Part model, mm, in its own coordinate system. A direction names the side the tool comes from. Give positions to 0.01 mm unless a question says otherwise; leave off trailing zeros. Write each loop counter-clockwise with the first axis right and the second up, starting at its lowest first coordinate (ties: lowest second). Pieces come first, ordered by that corner, then holes. Notation, with made-up numbers: (71.5, 53.5) - (98.5, 53.5) arc R26 ccw to (98.5, 89.5) - close; hole circle Ø3 at (-35, 15). An arc over 180 degrees is marked (long way). Answer in a Markdown table with one row per item. Add a question column.
1. Probe line 1 along Z through (x, y) = (-5.5, 11.5); line 2 along X through (y, z) = (11.5, 17.75); line 3 along X through (y, z) = (19, 14.5). List the from-to ranges inside material, lowest first.
2. Band-saw the part on A-A on x = 0. Write the cut outline in (y, z) (3 decimals), plus the area to 3 significant figures.
3. Pull direction Y, two halves, no side cores. Call faces 3 (the flat face through (-15.3, 45.4, 12.7)), 4 (the cylindrical face through (-37.794, -28.979, 15.831)), 5 (the flat face through (0, 0, 12.7)): released by +Y, released by -Y, zero draft, split by the parting line, or undercut.
4. Drop flat-ended pins along their axis: pin 1 Ø1.9 at (x, z) = (-4.5, 16) entering from -Y; pin 2 Ø6 at (x, z) = (-37, 10) entering from +Y; pin 3 Ø7 at (y, z) = (6.5, 16.5) entering from -X. Give the stop position or say it passes through.
5. Band-saw the part on C-C on z = 6.75. Write the cut outline in (x, y).
6. Band-saw the part on D-D on x = -28. Write the cut outline in (y, z), plus the area to 3 significant figures.
7. Which spindle directions (+Z, -Z, +X, -X, +Y, -Y) get a long thin tool onto all of the face, cutting with end or side? Do faces 1 (the flat face through (0, -19.05, 16)), 2 (the cylindrical face through (-11.012, -49.592, 6.261)). Say none if no direction does.
```python
from build123d import *

# Parameters (mm, degrees)
F0_R     = 50.8
F1_DEPTH = 12.7
F2_R     = 47.625
F3_DEPTH = 6.35
F4_W     = 38.1
F4_H     = 38.1
F5_DEPTH = 6.35


with BuildPart() as f1:
    # F0 (on Top) → F1 (new body)
    with BuildSketch(Plane.XY):
        Circle(F0_R)
    extrude(amount=F1_DEPTH)

    # F2 (on face) → F3 (join)
    with BuildSketch(Plane.XY.offset(12.7)):
        Circle(F2_R)
    extrude(amount=F3_DEPTH)

    # F4 (on face) → F5 (cut)
    with BuildSketch(Plane.XY.offset(19.05)):
        Rectangle(F4_W, F4_H)
    extrude(amount=-F5_DEPTH, mode=Mode.SUBTRACT)


solid = f1.part
```
Values:
| question | item | result |
|---|---|---|
| 1 | line 1 | z = 0 to 12.7 |
| 1 | line 2 | x = -46.22 to -19.05, 19.05 to 46.22 |
| 1 | line 3 | x = -43.67 to -19.05, 19.05 to 43.67 |
| 2 | outline | (-50.8, 0) - (50.8, 0) - (50.8, 12.7) - (47.625, 12.7) - (47.625, 19.05) - (19.05, 19.05) - (19.05, 12.7) - (-19.05, 12.7) - (-19.05, 19.05) - (-47.625, 19.05) - (-47.625, 12.7) - (-50.8, 12.7) - close |
| 2 | area | 1,650 mm² |
| 3 | face 3 | zero draft |
| 3 | face 4 | split by the parting line |
| 3 | face 5 | undercut |
| 4 | pin 1 | stops at y = -47.49 |
| 4 | pin 2 | stops at y = 37.74 |
| 4 | pin 3 | stops at x = -47.53 |
| 5 | outline | circle Ø101.6 at (0, 0) |
| 6 | outline | (-42.39, 0) - (42.39, 0) - (42.39, 12.7) - (38.52, 12.7) - (38.52, 19.05) - (-38.52, 19.05) - (-38.52, 12.7) - (-42.39, 12.7) - close |
| 6 | area | 1,570 mm² |
| 7 | face 1 | +Z |
| 7 | face 2 | +Z, -Z |
